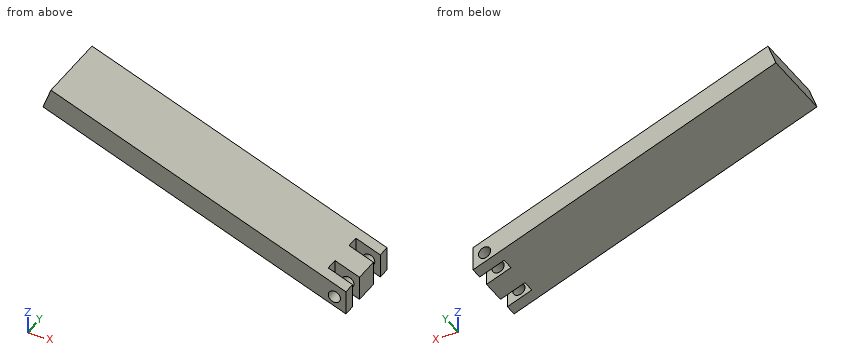
from build123d import *

# Parameters (mm, degrees)
F1_DEPTH = 38.1
F2_W     = 30.48
F2_H     = 12.699997
F3_DEPTH = 72.898
F4_R     = 6.35
F5_DEPTH = 38.1


with BuildPart() as f1:
    # F0 (on Front) → F1 (new body, symmetric)
    with BuildSketch(Plane.XZ):
        Polygon((190.276301, -36.691978), (-119.121099, 78.656576), (-127.435068, 56.356163), (190.276301, -62.091978), align=None)
    extrude(amount=F1_DEPTH, both=True)

    # F2 (on Top) → F3 (cut)
    with BuildSketch(Plane.XY):
        with Locations((179.884099, 19.347873)):
            Rectangle(F2_W, F2_H)
        with Locations((179.884092, -19.304001)):
            Rectangle(F2_W, F2_H)
    extrude(amount=-F3_DEPTH, mode=Mode.SUBTRACT)

    # F4 (on Front) → F5 (cut, symmetric)
    with BuildSketch(Plane.XZ):
        with Locations((178.126182, -46.895169)):
            Circle(F4_R)
    extrude(amount=F5_DEPTH, both=True, mode=Mode.SUBTRACT)


with BuildPart() as f1_1:
    # F6: moved
    add(f1.part.moved(Location((-31.496, 0, -8.636))))


solid = f1_1.part
Could you check a few things on this model? Use its own coordinates, in mm. Coordinates: 2 decimals unless noted, no trailing zeros. Write each loop counter-clockwise with the first axis right and the second up, starting at its lowest first coordinate (ties: lowest second). Pieces come first, ordered by that corner, then holes. Notation, with made-up numbers: (6.25, -28) - (13.25, -28) arc R15 cw to (13.25, 0) - close; hole circle Ø10 at (41, 57.5). An arc over 180 degrees is marked (long way). Write item = value, one per line.
1) Suppose I cut it at B-B on y = -9.5. Please give me the cut outline in (x, z), plus the area to 3 significant figures.
Result set:
outline = (-158.93, 47.72) - (158.78, -70.73) - (158.78, -45.33) - (-150.62, 70.02) - close; hole circle Ø12.7 at (146.63, -55.53)
area = 7,840 mm2
2) Suppose I cut it at A-A on y = 18.5. Please give me the cut outline in (x, z), plus the area to 3 significant figures.
Result set:
outline = (-158.93, 47.72) - (133.15, -61.17) - (133.15, -35.77) - (-150.62, 70.02) - close
area = 7,310 mm2
3) Will these pins go through, and if not, where does the flat tip stop? pin 1 Ø8 at (x, y) = (-76.5, 5.5) entering from +Z; pin 2 Ø4 at (y, z) = (-16.5, -47) entering from +X; pin 3 Ø10 at (x, z) = (146.63, -55.53) entering from -Y; pin 4 Ø8 at (y, z) = (-27.5, 44.5) entering from -X.
Result set:
pin_1 = 43.88
pin_2 = 133.15
pin_3 = through
pin_4 = -158.93
4) Please list where these lines run through material, in increasing order: line 1 (Z direction, x = 116, y = 28); line 2 (Z direction, x = -61.5, y = -7.5). Write a range as [from, to].
Result set:
line_1 = [-54.78, -29.38]
line_2 = [11.4, 36.8]
5) Suppose I cut it at C-C on x = 122.5. Please give me the cut outline in (y, z), plus the area to 3 significant figures.
Result set:
outline = (-38.1, -57.2) - (38.1, -57.2) - (38.1, -31.8) - (-38.1, -31.8) - close
area = 1,940 mm2
